```python
from build123d import *

# Parameters (mm, degrees)
SKETCH1_W               = 31.999999976
SKETCH1_H               = 4
BOSS_EXTRUDE1_DEPTH     = 5
SKETCH2_W               = 2.499999921
SKETCH2_H               = 4
BOSS_EXTRUDE2_DEPTH     = 3
SKETCH3_W               = 2.999999921
SKETCH3_H               = 4
BOSS_EXTRUDE3_DEPTH     = 2
CIRPATTERN1_COUNT       = 2
CIRPATTERN1_ANGLE       = 90
CUT_EXTRUDE1_DEPTH      = 3.250000112
BOSS_EXTRUDE4_DEPTH     = 1
CUT_EXTRUDE_THIN1_START = -3.25
CUT_EXTRUDE_THIN1_DEPTH = 3.25
CUT_EXTRUDE_THIN2_START = -3.25
CUT_EXTRUDE_THIN2_DEPTH = 3.25
CHAMFER2_SIZE           = 1
CHAMFER3_SIZE           = 0.4


with BuildPart() as part:
    # Sketch1 → Boss-Extrude1 (new body)
    with BuildSketch(Plane(origin=(0, 0, 0), x_dir=(1, 0, 0), z_dir=(0, 1, 0))):
        Rectangle(SKETCH1_W, SKETCH1_H)
    extrude(amount=BOSS_EXTRUDE1_DEPTH)

    # Sketch2 → Boss-Extrude2 (add)
    with BuildSketch(Plane.XZ):
        with Locations((14.750000028, 0)):
            Rectangle(SKETCH2_W, SKETCH2_H)
        with Locations((-14.750000028, 0)):
            Rectangle(SKETCH2_W, SKETCH2_H)
    extrude(amount=BOSS_EXTRUDE2_DEPTH)

    # Sketch3 → Boss-Extrude3 (add)
    with BuildSketch(Plane.XZ.offset(3)):
        with Locations((14.500000028, 0)):
            Rectangle(SKETCH3_W, SKETCH3_H)
        with Locations((-14.500000028, 0)):
            Rectangle(SKETCH3_W, SKETCH3_H)
    extrude(amount=BOSS_EXTRUDE3_DEPTH)

    # CirPattern1: part ×2 about axis
    cirpattern1_axis = Axis((0, 0, 0), (0, 1, 0))


with BuildPart() as part_1:
    add(part.part)
    for i in range(1, CIRPATTERN1_COUNT):
        add(part.part.rotate(cirpattern1_axis, i * CIRPATTERN1_ANGLE / (CIRPATTERN1_COUNT - 1)))

    # Sketch6 → Cut-Extrude1 (cut)
    with BuildSketch(Plane(origin=(0, 5, 0), x_dir=(1, 0, 0), z_dir=(0, 1, 0))):
        Polygon((-1.414213562, -9.545941546), (-9.545941546, -1.414213562), (1.414213562, 9.545941546), (6.01040764, 4.949747468), (4.949747468, 3.889087297), (8.485281374, 0.353553391), align=None)
    extrude(amount=-CUT_EXTRUDE1_DEPTH, mode=Mode.SUBTRACT)

    # Sketch7 → Boss-Extrude4 (add)
    with BuildSketch(Plane(origin=(0, 5, 0), x_dir=(1, 0, 0), z_dir=(0, 1, 0))):
        Polygon((-9.545941546, -1.414213562), (-9.192388155, -1.767766953), (-5.424621202, 2), (-6.131727984, 2), align=None)
        Polygon((1.767766953, 9.192388155), (1.414213562, 9.545941546), (-2, 6.131727984), (-2, 5.424621202), align=None)
        Polygon((8.131727984, 0.707106781), (8.485281374, 0.353553391), (6.131727984, -2), (5.424621202, -2), align=None)
        Polygon((2, -5.424621202), (2, -6.131727984), (-1.414213562, -9.545941546), (-1.767766953, -9.192388155), align=None)
    extrude(amount=-BOSS_EXTRUDE4_DEPTH)

    # Sketch8 → Cut-Extrude-Thin1 (cut)
    with BuildSketch(Plane(origin=(0, 5, 0), x_dir=(1, 0, 0), z_dir=(0, 1, 0)).offset(CUT_EXTRUDE_THIN1_START)):
        Polygon((-9.424621202, -2), (2, 9.424621202), (3.796051224, 7.628569978), (-7.628569978, -3.796051224), align=None)
    extrude(amount=CUT_EXTRUDE_THIN1_DEPTH, mode=Mode.SUBTRACT)

    # Sketch9 → Cut-Extrude-Thin2 (cut)
    with BuildSketch(Plane(origin=(0, 5, 0), x_dir=(1, 0, 0), z_dir=(0, 1, 0)).offset(CUT_EXTRUDE_THIN2_START)):
        Polygon((2, -5.424621202), (-2, -9.424621202), (-3.796051224, -7.628569978), (0.203948776, -3.628569978), align=None)
    extrude(amount=CUT_EXTRUDE_THIN2_DEPTH, mode=Mode.SUBTRACT)

    # Chamfer2
    chamfer2_edges = [part_1.edges().sort_by_distance(p)[0] for p in [
        (0, 0, 13.500000067),
        (0, -5, -13.000000067),
        (0, -5, 13.000000067),
        (13.500000067, 0, 0),
        (-13.500000067, 0, 0),
        (13.000000067, -5, 0),
        (-13.000000067, -5, 0),
        (0, 0, -13.500000067),
    ]]
    chamfer(chamfer2_edges, length=CHAMFER2_SIZE)

    # Chamfer3
    chamfer3_edges = [part_1.edges().sort_by_distance(p)[0] for p in [
        (15.999999988, 5, 0),
        (0, -5, -15.999999988),
        (0, -5, 15.999999988),
        (11.419417376, 5, -2),
        (10.712310595, 5, 2),
        (-10.712310595, 5, -2),
        (-7.424621202, 5, 0),
        (0, 5, -7.424621202),
        (7.485281374, 5, -1.353553391),
        (6.778174593, 5, 0.646446609),
        (0, 5, 7.424621202),
        (2, 5, -12.712310595),
        (-2, 5, 12.712310595),
        (15.999999988, -5, 0),
        (-15.999999988, 5, 0),
        (-15.999999988, -5, 0),
        (-12.712310595, 5, 2),
        (0, 5, 15.999999988),
        (2, 5, 10.712310595),
        (0, 5, -15.999999988),
        (-2, 5, -10.712310595),
        (2, 0, 15.999999988),
        (-2, 0, -15.999999988),
        (-15.999999988, 0, -2),
        (-2, 0, 15.999999988),
        (2, 0, -15.999999988),
        (15.999999988, 0, -2),
        (15.999999988, 0, 2),
        (-15.999999988, 0, 2),
    ]]
    chamfer(chamfer3_edges, length=CHAMFER3_SIZE)


solid = part_1.part
```
The listing builds one solid part. Answer for the finished solid, in the listing's coordinates (mm). A direction names the side the tool comes from. Give positions to 0.01 mm unless a question says otherwise; leave off trailing zeros. Order: outer loops, then holes, each group sorted by start corner. A loop starts at its lowest first (then second) coordinate and runs counter-clockwise, first axis right, second up.
1) Determine the mould class of faces 6 (the face through (-13, -3.5, 0)), 7 (the face through (16, 0, 0)), 8 (the face through (0, 0, 16)) for opening direction X: pulls with the +X half, pulls with the -X half, needs draft (parallel to the pull), parting line crosses it, or undercut.
Reported:
face 6: undercut
face 7: pulls with the +X half
face 8: needs draft
2) Given P1, Ø5.5, axis at x = -4.5, z = 4, coming from the +Y side; P2, Ø3, axis at x = 12, y = -1.5, coming from the -Z side; P3, Ø1, axis at x = -7.5, z = 2, coming from the -Y side; P4, Ø1.5, axis at y = -1.5, z = 6, coming from the -X side, each flat-ended and moving along its own axis, determine where each tip first touches the part or whether it passes through.
Reported:
P1: stops at y = 1.75
P2: stops at z = -2
P3: stops at y = 0
P4: passes through
3) Find section B-B on x = -12. Write down the section's boundary in (y, z), then the cut area to 3 significant figures.
Reported:
outline: (0, -2) - (4.6, -2) - (5, -1.6) - (5, 1.6) - (4.6, 2) - (0, 2) - close
area: 19.8 mm2
4) Find section A-A on y = -1.5. Write down the section's boundary in (x, z).
Reported:
outline: (-16, -1.6) - (-15.6, -2) - (-13.5, -2) - (-13.5, 2) - (-15.6, 2) - (-16, 1.6) - close; (-2, -15.6) - (-1.6, -16) - (1.6, -16) - (2, -15.6) - (2, -13.5) - (-2, -13.5) - close; (-2, 13.5) - (2, 13.5) - (2, 15.6) - (1.6, 16) - (-1.6, 16) - (-2, 15.6) - close; (13.5, -2) - (15.6, -2) - (16, -1.6) - (16, 1.6) - (15.6, 2) - (13.5, 2) - close
5) For faces 1 (the face through (-13, -0.5, 0)), 2 (the face through (-0.17, 4.8, -7.54)), 3 (the face through (0, -0.5, -13)), 4 (the face through (-0.287, 4.224, 7.712)), 5 (the face through (2, 1, 10)), determine the directions among +Z, -Z, +X, -X, +Y, -Y from which every point of the face is accessible in a straight line to the end or side of a thin tool.
Reported:
face 1: +Z, -Z
face 2: +X, +Y
face 3: +X, -X
face 4: -X, +Y
face 5: +Z, +X, +Y, -Y
6) Find section C-C on z = 10. Write down the section's boundary in (x, y).
Reported:
outline: (-2, 0) - (2, 0) - (2, 4.6) - (1.6, 5) - (-1.6, 5) - (-2, 4.6) - close
7) Find section D-D on y = 3.25. Give the number of separate pieces and of enclosed holes in the cut face, then the cut area to 3 significant figures.
Reported:
separate pieces: 4
enclosed holes: 0
area: 129 mm2
8) Consider line 1 along X through (y, z) = (-3.75, 0); line 2 along X through (y, z) = (3, 11). Determine where each line is inside the solid, lowest interval first.
Reported:
line 1: x = -16 to -13, 13 to 16
line 2: x = -2 to 2
